from build123d import *

# Parameters (mm, degrees)
SKETCH1_W                = 21.5
SKETCH1_H                = 21.5
BOSS_EXTRUDE1_DEPTH      = 0.5
SKETCH2_R                = 2.3
SKETCH2_W                = 4
SKETCH2_H                = 4
SKETCH2_H_2              = 7
SKETCH2_W_2              = 7
CUT_EXTRUDE1_DEPTH       = 1.5
FILLET1_R                = 2
SKETCH3_W                = 0.6
SKETCH3_H                = 10.5
SKETCH3_W_2              = 10.5
SKETCH3_H_2              = 0.6
BOSS_EXTRUDE2_DEPTH      = 4.5
BOSS_EXTRUDE2_DEPTH_BACK = 0.5
FILLET11_R               = 0.5
SKETCH6_W                = 15
SKETCH6_H                = 0.5
BOSS_EXTRUDE3_DEPTH      = 1.2
BOSS_EXTRUDE4_DEPTH      = 2
SKETCH9_W                = 15
SKETCH9_H                = 0.5
BOSS_EXTRUDE5_DEPTH      = 4
FILLET12_R               = 0.5
FILLET13_R               = 2


with BuildPart() as part:
    # Sketch1 → Boss-Extrude1 (new body)
    with BuildSketch(Plane(origin=(0, 0, 0), x_dir=(1, 0, 0), z_dir=(0, 1, 0))):
        with Locations((10.75, 10.75)):
            Rectangle(SKETCH1_W, SKETCH1_H)
    extrude(amount=BOSS_EXTRUDE1_DEPTH)

    # Sketch2 → Cut-Extrude1 (cut, through all)
    with BuildSketch(Plane(origin=(0, 0.5, 0), x_dir=(1, 0, 0), z_dir=(0, 1, 0))):
        Polygon((0, 21.5), (21.5, 0), (0, 0), align=None)
        with Locations((13.88, 13.88)):
            Circle(SKETCH2_R)
        with Locations((19.5, 19.5)):
            Rectangle(SKETCH2_W, SKETCH2_H)
        with Locations((19.5, 14)):
            Rectangle(SKETCH2_W, SKETCH2_H_2)
        with Locations((14, 19.5)):
            Rectangle(SKETCH2_W_2, SKETCH2_H)
    extrude(amount=-CUT_EXTRUDE1_DEPTH, mode=Mode.SUBTRACT)

    # Fillet1
    fillet1_edges = [part.edges().sort_by_distance(p)[0] for p in [
        (17.5, 0.25, -17.5),
    ]]
    fillet(fillet1_edges, radius=FILLET1_R)

    # Sketch3 → Boss-Extrude2 (add, two sides)
    with BuildSketch(Plane(origin=(0, 0.5, 0), x_dir=(1, 0, 0), z_dir=(0, 1, 0))) as boss_extrude2_sk:
        with Locations((21.2, 5.25)):
            Rectangle(SKETCH3_W, SKETCH3_H)
        with Locations((5.25, 21.2)):
            Rectangle(SKETCH3_W_2, SKETCH3_H_2)
    extrude(amount=BOSS_EXTRUDE2_DEPTH)
    extrude(boss_extrude2_sk.sketch, amount=-BOSS_EXTRUDE2_DEPTH_BACK)

    # Fillet11
    fillet11_edges = [part.edges().sort_by_distance(p)[0] for p in [
        (5.25, 0, -21.5),
        (21.5, 0, -5.25),
        (20.9, 0.5, -5.55),
        (21.2, 5, -10.5),
        (21.2, 5, 0),
        (5.55, 0.5, -20.9),
        (10.5, 5, -21.2),
        (0, 5, -21.2),
    ]]
    fillet(fillet11_edges, radius=FILLET11_R)

    # Sketch6 → Boss-Extrude3 (add)
    with BuildSketch(Plane(origin=(10.75, 0, -10.75), x_dir=(0.707106781, 0, 0.707106781), z_dir=(-0.707106781, 0, 0.707106781))):
        with Locations((0, 0.25)):
            Rectangle(SKETCH6_W, SKETCH6_H)
    extrude(amount=BOSS_EXTRUDE3_DEPTH)

    # Sketch8 → Boss-Extrude4 (add)
    with BuildSketch(Plane.XZ):
        Polygon((4.598171004, -15.204772721), (15.204772721, -4.598171004), (15.62903679, -5.022435072), (5.022435072, -15.62903679), align=None)
    extrude(amount=BOSS_EXTRUDE4_DEPTH)

    # Sketch9 → Boss-Extrude5 (add)
    with BuildSketch(Plane(origin=(9.901471863, 0, -9.901471863), x_dir=(0.707106781, 0, 0.707106781), z_dir=(-0.707106781, 0, 0.707106781))):
        with Locations((0, -1.75)):
            Rectangle(SKETCH9_W, SKETCH9_H)
    extrude(amount=BOSS_EXTRUDE5_DEPTH)

    # Fillet12
    fillet12_edges = [part.edges().sort_by_distance(p)[0] for p in [
        (9.901471863, 0.5, -9.901471863),
        (10.325735931, 0, -10.325735931),
        (10.325735931, -2, -10.325735931),
        (9.901471863, -1.5, -9.901471863),
    ]]
    fillet(fillet12_edges, radius=FILLET12_R)

    # Fillet13
    fillet13_edges = [part.edges().sort_by_distance(p)[0] for p in [
        (1.769743879, -1.75, -12.376345597),
        (12.376345597, -1.75, -1.769743879),
    ]]
    fillet(fillet13_edges, radius=FILLET13_R)


solid = part.part
Part model, mm, in its own coordinate system. A direction names the side the tool comes from. Coordinates: 2 decimals unless noted, no trailing zeros. Loops run counter-clockwise (first coordinate to the right, second up) from the corner with the lowest first, then second, coordinate; pieces in that order, holes last. Notation, with made-up numbers: (73, 8.5) - (103, 8.5) arc R24 ccw to (103, 31.5) - close; hole circle Ø10 at (64, -1). An arc over 180 degrees is marked (long way). Write each question's results on one line, items separated by ' | '. Start each with the question number.
Q1. Probe line 1 along Z through (x, y) = (4.25, 4); line 2 along X through (y, z) = (0.3, -13.88); line 3 along X through (y, z) = (0.2, -13.88). List the from-to ranges inside material, lowest first.
Q2. Slice it at A-A on y = 3.75. Give the cut face in (x, z).
Q3. Two-plate mould, pull along Z, no slides. Class faces 1 (the flat face through (10.5, 1.6, -21.1)), 2 (the cylindrical face through (12.055, 0.254, -12.48)), 3 (the cylindrical face through (10.145, -1.857, -10.294)): +Z half, -Z half, draft (parallel to the pull), parting line (faces both ways), or undercut.
Q4. Which spindle directions (+Z, -Z, +X, -X, +Y, -Y) get a long thin tool onto all of the face, cutting with end or side? Do faces 4 (the flat face through (12, 0, -12)), 5 (the flat face through (21.1, 1.4, -10.5)), 6 (the flat face through (8, -1.5, -8)). Say none if no direction does.
Q5. Drop flat-ended pins along their axis: pin 1 Ø6 at (x, z) = (13.88, -13.88) entering from +Y; pin 2 Ø2 at (y, z) = (1, -18.5) entering from +X; pin 3 Ø2 at (x, z) = (7.5, -5.5) entering from +Y. Give the stop position or say it passes through.
Q6. Slice it at B-B on z = -16.75. Give the cut face in (x, y), and give its area (3 significant figures).
Answer:
1) line 1: z = -21.5 to -20.9 | line 2: x = 6.06 to 11.58, 16.18 to 17.5 | line 3: x = 5.98 to 11.58, 16.18 to 17.5
2) outline: (0, -21.5) - (10.5, -21.5) - (10.5, -20.9) - (0, -20.9) - close; (20.9, -10.5) - (21.5, -10.5) - (21.5, 0) - (20.9, 0) - close
3) face 1: draft | face 2: undercut | face 3: -Z half
4) face 4: -Z, +X, -Y | face 5: -Z, +X, +Y, -Y | face 6: +Z, -X, +Y
5) pin 1: stops at y = 0.5 | pin 2: stops at x = 10.5 | pin 3: stops at y = -1.5
6) outline: (4.75, 0) - (17.06, 0) - (17.06, 0.5) - (4.75, 0.5) - close | area: 6.16 mm2
